```python
from build123d import *

# Parameters (mm, degrees)
SKETCH1_R           = 7.5
SKETCH1_R_2         = 3.5
SKETCH1_R_3         = 2.375
BOSS_EXTRUDE1_DEPTH = 2.5
SKETCH1_3_R         = 2.375
BOSS_EXTRUDE2_DEPTH = 120
BOSS_EXTRUDE3_START = -75
SKETCH1_4_R         = 3.5
SKETCH1_4_R_2       = 2.375
BOSS_EXTRUDE3_DEPTH = 20
FILLET1_R           = 2


with BuildPart() as part:
    # Sketch1 → Boss-Extrude1 (new body)
    with BuildSketch(Plane.XY):
        Circle(SKETCH1_R)
        Circle(SKETCH1_R_2, mode=Mode.SUBTRACT)
        Circle(SKETCH1_R_2)
        Circle(SKETCH1_R_3, mode=Mode.SUBTRACT)
        Circle(SKETCH1_R_3)
    extrude(amount=BOSS_EXTRUDE1_DEPTH)

    # Sketch1_3 → Boss-Extrude2 (add)
    with BuildSketch(Plane.XY):
        Circle(SKETCH1_3_R)
    extrude(amount=-BOSS_EXTRUDE2_DEPTH)

    # Sketch1_4 → Boss-Extrude3 (add)
    with BuildSketch(Plane.XY.offset(BOSS_EXTRUDE3_START)):
        Circle(SKETCH1_4_R)
        Circle(SKETCH1_4_R_2, mode=Mode.SUBTRACT)
    extrude(amount=-BOSS_EXTRUDE3_DEPTH)

    # Fillet1
    fillet1_edges = [part.edges().sort_by_distance(p)[0] for p in [
        (-7.5, 0, 2.5),
    ]]
    fillet(fillet1_edges, radius=FILLET1_R)


solid = part.part
```
Check sheet for the modelled part. Datum: model origin and axes. Units: mm. A direction names the side the tool comes from. Round coordinates to 2 decimals unless told otherwise and drop trailing zeros. Write each loop counter-clockwise with the first axis right and the second up, starting at its lowest first coordinate (ties: lowest second). Pieces come first, ordered by that corner, then holes. Notation, with made-up numbers: M -5.5,1 L 37.5,1 A28 ccw 37.5,33 Z; hole C 9,78 d2. An arc over 180 degrees is marked long. Write item = value, one per line. Start each with the question number.
1. Release check for a two-part mould opening along Z. For faces 1 (the flat face through (0, 0, -120)), 2 (the cylindrical face through (1.096, -2.107, -36.975)), 3 (the cylindrical face through (1.096, -2.107, -107.325)) record: pulls with the +Z half, pulls with the -Z half, needs draft (parallel to the pull), parting line crosses it, or undercut.
2. Section check C-C, the plane z = -102.5. Record the cut outline in (x, y) (3 decimals).
3. Tool access check on faces 4 (the cylindrical face through (3.233, -1.341, -84.86)), 5 (the flat face through (0, 0, 2.5)). Record the directions out of +Z, -Z, +X, -X, +Y, -Y that give a thin tool (end or side, any length) a straight path to the whole face; none if there is none.
4. Gauge pin test, flat ends, axial feed: pin 1 (4 mm diameter, centred on x = 2.5, z = -51, fed in from +Y); pin 2 (3 mm diameter, centred on x = 0, y = -4, fed in from -Z); pin 3 (2 mm diameter, centred on x = 6, y = 2.5, fed in from -Z). Record the tip position at first contact, or that the pin passes through.
5. Section check A-A, the plane x = 0. Record the cut outline in (y, z) (3 decimals), then the cut area to 3 significant figures.
6. Scan lines: line 1 (Z direction, x = 1.5, y = -2.5); line 2 (Z direction, x = -3.5, y = 1); line 3 (Y direction, x = -0.25, z = -49.5). Record each from-to range of solid material in increasing order. Write a range as [from, to].
Results found:
q1.face_1 = pulls with the -Z half
q1.face_2 = undercut
q1.face_3 = needs draft
q2.outline = C 0,0 d4.75
q3.face_4 = -Z
q3.face_5 = +Z, +X, -X, +Y, -Y
q4.pin_1 = 2.32
q4.pin_2 = -95
q4.pin_3 = 0
q5.outline = M -7.5,0 L -2.375,0 L -2.375,-75 L -3.5,-75 L -3.5,-95 L -2.375,-95 L -2.375,-120 L 2.375,-120 L 2.375,-95 L 3.5,-95 L 3.5,-75 L 2.375,-75 L 2.375,0 L 7.5,0 L 7.5,0.5 A2 ccw 5.5,2.5 L -5.5,2.5 A2 ccw -7.5,0.5 Z
q5.area = 651 mm^2
q6.line_1 = [-95, -75], [0, 2.5]
q6.line_2 = [0, 2.5]
q6.line_3 = [-2.36, 2.36]
